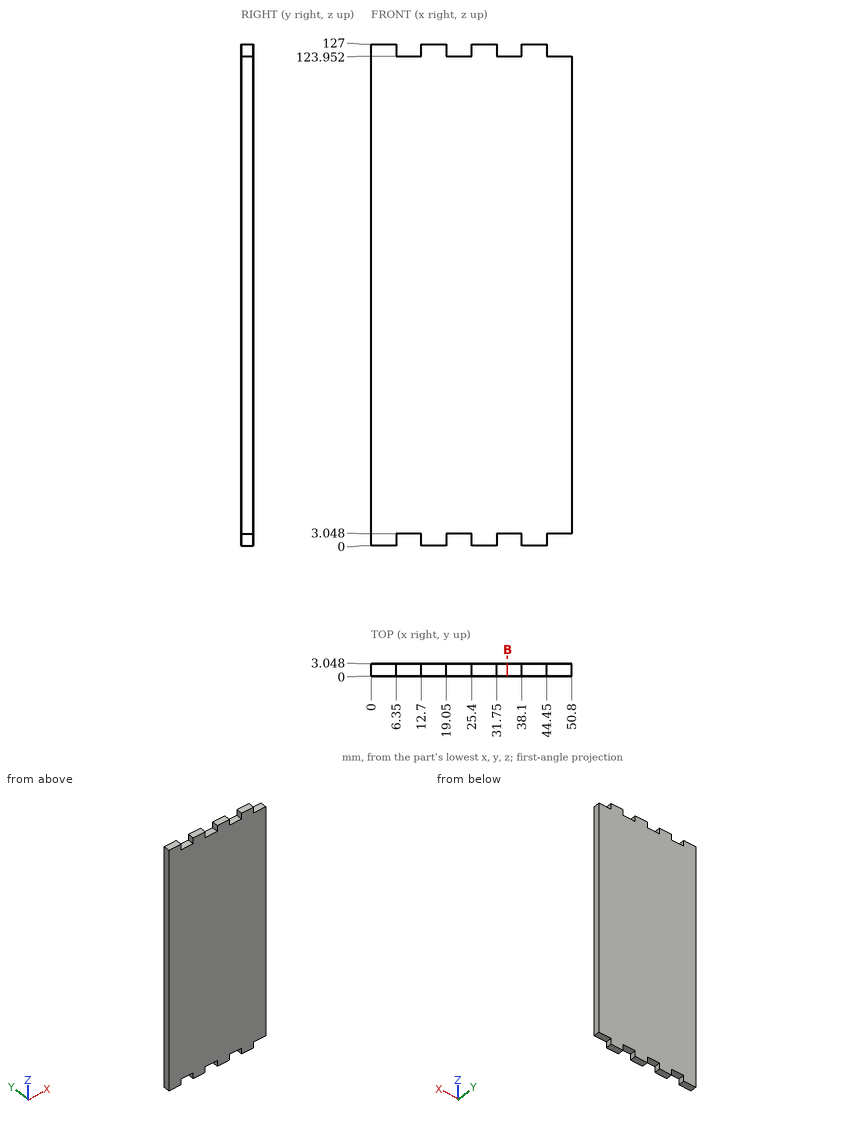
Geometry check sheet. Reference: drawing and pictorial views, mm from the part's lowest x, y, z. Give positions to 0.01 mm unless a question says otherwise; leave off trailing zeros. Loops run counter-clockwise (first coordinate to the right, second up) from the corner with the lowest first, then second, coordinate; pieces in that order, holes last. Notation, with made-up numbers: (26.25, -26) - (53.25, -26) arc R19 cw to (53.25, 9) - close; hole circle Ø9 at (53.5, -15.75). An arc over 180 degrees is marked (long way). Use CSV: the item, a comma, the result in double quotes. Start each with the question number.
Q1. Section check B-B, the plane x = 34.5. Record the cut outline in (y, z).
Q2. Go/stop test with flat-tipped pins: pin 1 Ø0.9 at (y, z) = (2, 2) entering from +X; pin 2 Ø0.9 at (x, y) = (8.5, 1.5) entering from -Z; pin 3 Ø1.5 at (x, y) = (36, 1.5) entering from +Z. Record where each tip stops, or that it passes through.
Q3. Scan line: probe 1 along Z at (x, y) = (37.5, 0.8). Record every from-to range of solid material in increasing order. Write a range as from..to.
Findings below:
1,outline,"(0, 3.05) - (3.05, 3.05) - (3.05, 123.95) - (0, 123.95) - close"
2,pin 1,"stops at x = 44.45"
2,pin 2,"stops at z = 3.05"
2,pin 3,"stops at z = 123.95"
3,probe 1,"z = 3.05..123.95"
